Source: three-view drawing plus pictorial views. Frame: mm from the lowest corner of the part. A direction names the side the tool comes from. Give positions to 0.01 mm unless a question says otherwise; leave off trailing zeros. Loops run counter-clockwise (first coordinate to the right, second up) from the corner with the lowest first, then second, coordinate; pieces in that order, holes last.
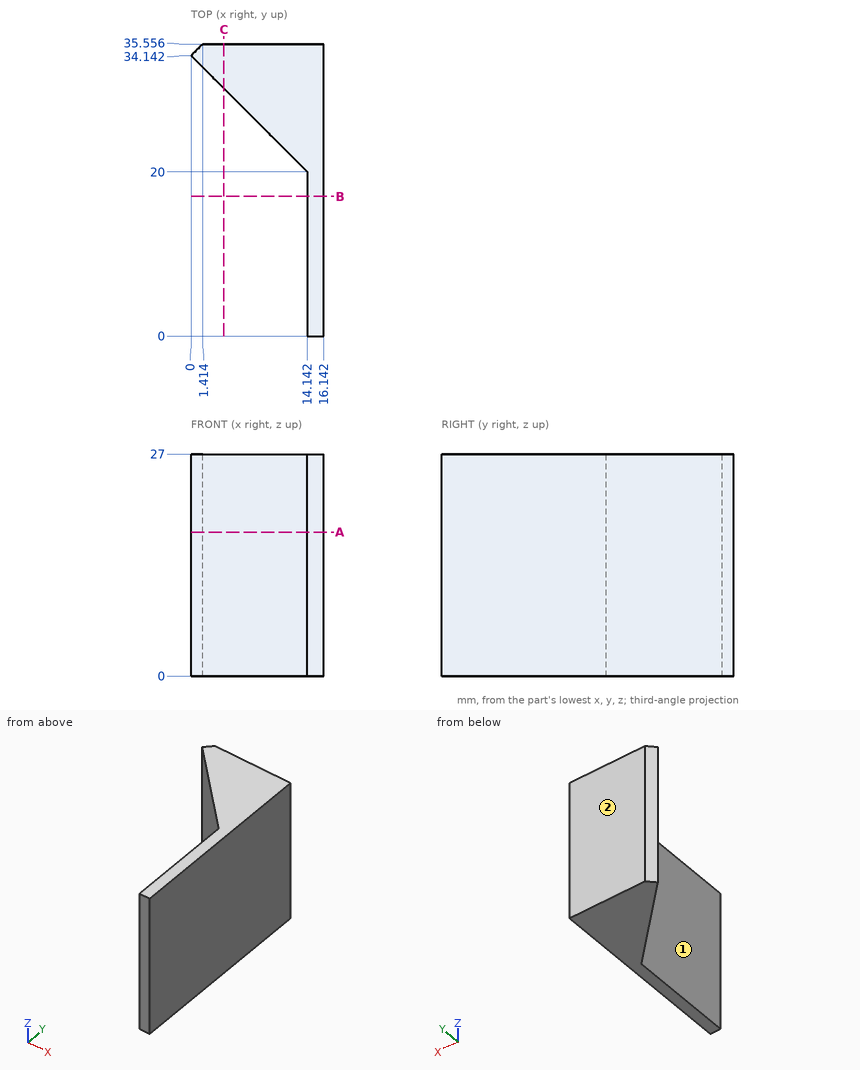
(1) Reachability of the marked faces 1 and 2 from +Z, -Z, +X, -X, +Y, -Y: full face, straight path, thin tool, end or side. Return the list, or none.
Values follow:
face 1: +Z, -Z, -X, -Y
face 2: +Z, -Z, +X, -X, +Y
(2) Cut plane C-C (x = 4). Return the cut outline in (y, z), and give its area (3 significant figures).
Values follow:
outline: (30.14, 0) - (35.56, 0) - (35.56, 27) - (30.14, 27) - close
area: 146 mm2
(3) Pin query (flat end, axial travel): pin 1 Ø1.5 at (y, z) = (30.5, 15.5) entering from -X; pin 2 Ø2 at (y, z) = (6, 15) entering from -X; pin 3 Ø1.5 at (y, z) = (20.5, 15) entering from -X. Return the tip coordinate at first contact, or that it passes through.
Values follow:
pin 1: stops at x = 2.89
pin 2: stops at x = 14.14
pin 3: stops at x = 12.89
(4) Cut plane A-A (z = 17.5). Return the cut outline in (x, y).
Values follow:
outline: (0, 34.14) - (14.14, 20) - (14.14, 0) - (16.14, 0) - (16.14, 35.56) - (1.41, 35.56) - close
(5) Ray query, probe 1 along X at (y, z) = (15.5, 6.5); probe 2 along X at (y, z) = (32, 7.25); probe 3 along Y at (x, z) = (10.5, 8.5) (1 decimal). Return the intervals inside material, ascending.
Values follow:
probe 1: x = 14.14 to 16.14
probe 2: x = 2.14 to 16.14
probe 3: y = 23.6 to 35.6
(6) Cut plane B-B (y = 17). Return the cut outline in (x, z).
Values follow:
outline: (14.14, 0) - (16.14, 0) - (16.14, 27) - (14.14, 27) - close
